Model file for the job. Use its own axes, mm. A direction names the side the tool comes from. Give positions to 0.01 mm unless a question says otherwise; leave off trailing zeros. Write each loop counter-clockwise with the first axis right and the second up, starting at its lowest first coordinate (ties: lowest second). Pieces come first, ordered by that corner, then holes. Notation, with made-up numbers: (1, 75.5) - (5, 75.5) arc R11 ccw to (5, 94.5) - close; hole circle Ø8 at (6, 70.25). An arc over 180 degrees is marked (long way). One line per item, written item: value. Start each with the question number.
(1) Cut at D-D, the plane z = -4.5. List the corners of the cut face in (x, y), and give its area (3 significant figures).
(2) 3-axis set-ups, long thin cutter, end or side, ignore diameter. For faces 1 (the face through (2.957, -0.931, -6.827)), 2 (the face through (-6, 9, -7)), 3 (the face through (-0.553, -4.214, -2.535)): which of +Z, -Z, +X, -X, +Y, -Y reach the whole face in a straight line?
(3) Cut at C-C, the plane z = -6.5. List the corners of the cut face in (x, y).
(4) Mould opens along X. For faces 4 (the face through (11.923, -3.755, -6.26)), 5 (the face through (-4, 2, -8.2)), 6 (the face through (-0.74, 3.32, -2.56)) say: pulls with the +X half, pulls with the -X half, needs draft (parallel to the pull), parting line crosses it, or undercut.
(5) Probe L1, parallel to Y at x = 0, z = -6.5; L2, parallel to Y at x = 0, z = -2.4; L3, parallel to Y at x = 0, z = -5.9. List the from-to ranges inside material, lowest first.
(6) Drop flat-ended pins along their axis: P1, Ø2, axis at x = 0.5, y = 1, coming from the +Z side; P2, Ø6, axis at x = 4.5, y = 7, coming from the +Z side; P3, Ø3, axis at y = 6, z = -5.5, coming from the -X side; P4, Ø3, axis at y = -4.5, z = -5.5, coming from the +X side. Give the stop position or say it passes through.
from build123d import *

# Parameters (mm, degrees)
CHAMFER1_SIZE = 0.5


with BuildPart() as part:
    # Sketch1 → Revolve1 (revolve)
    with BuildSketch(Plane(origin=(0, 0, 0), x_dir=(0, 0, -1), z_dir=(1, 0, 0)), mode=Mode.PRIVATE) as revolve1_sk:
        Polygon((0, 3.4), (0, 4.25), (5, 4.25), (5, 12.5), (7, 12.5), (7, 10.6), (6, 10.6), (6, 7.9), (7, 7.9), (7, 4.75), (8.2, 4.75), (8.2, 4), (8.5, 4), (8.5, 3.1), (5.2, 3.1), (5.2, 3.4), align=None)
    revolve(revolve1_sk.sketch.rotate(Axis((0, 0, 0), (0, 0, -1)), 90), axis=Axis((0, 0, 0), (0, 0, -1)))

    # Chamfer1
    chamfer1_edges = [part.edges().sort_by_distance(p)[0] for p in [
        (-12.5, 0, -5),
    ]]
    chamfer(chamfer1_edges, length=CHAMFER1_SIZE)


solid = part.part
Answers follow:
1. outline: circle Ø8.5 at (0, 0); hole circle Ø6.8 at (0, 0)
1. area: 20.4 mm²
2. face 1: +Z, -Z
2. face 2: -Z
2. face 3: +Z
3. outline: circle Ø25 at (0, 0); circle Ø15.8 at (0, 0); hole circle Ø21.2 at (0, 0); hole circle Ø6.2 at (0, 0)
4. face 4: parting line crosses it
4. face 5: needs draft
4. face 6: undercut
5. L1: y = -12.5 to -10.6, -7.9 to -3.1, 3.1 to 7.9, 10.6 to 12.5
5. L2: y = -4.25 to -3.4, 3.4 to 4.25
5. L3: y = -12.5 to -3.1, 3.1 to 12.5
6. P1: passes through
6. P2: stops at z = -5
6. P3: stops at x = -11.66
6. P4: stops at x = 12.13
